```python
from build123d import *

# Parameters (mm, degrees)
SKETCH1_R           = 8
BOSS_EXTRUDE1_DEPTH = 6
SKETCH2_R           = 9.5
BOSS_EXTRUDE2_DEPTH = 2
SKETCH3_R           = 6.25
SKETCH3_R_2         = 4.25
CUT_EXTRUDE1_DEPTH  = 5
CHAMFER1_SIZE       = 1
CHAMFER2_SIZE       = 1
CUT_EXTRUDE2_DEPTH  = 16.636495771
CUT_EXTRUDE3_DEPTH  = 0.5


with BuildPart() as part:
    # Sketch1 → Boss-Extrude1 (new body)
    with BuildSketch(Plane(origin=(0, 0, 0), x_dir=(1, 0, 0), z_dir=(0, 1, 0))):
        with Locations(Location((0, 0, 0), (0, 0, 270))):
            Circle(SKETCH1_R)
    extrude(amount=BOSS_EXTRUDE1_DEPTH)

    # Sketch2 → Boss-Extrude2 (add)
    with BuildSketch(Plane.XZ):
        with Locations(Location((0, 0, 0), (0, 0, 270))):
            Circle(SKETCH2_R)
    extrude(amount=BOSS_EXTRUDE2_DEPTH)

    # Sketch3 → Cut-Extrude1 (cut)
    with BuildSketch(Plane.XZ.offset(2)):
        with Locations(Location((0, 0, 0), (0, 0, 270))):
            Circle(SKETCH3_R)
        with Locations(Location((0, 0, 0), (0, 0, 270))):
            Circle(SKETCH3_R_2, mode=Mode.SUBTRACT)
    extrude(amount=-CUT_EXTRUDE1_DEPTH, mode=Mode.SUBTRACT)

    # Chamfer1
    chamfer1_edges = [part.edges().sort_by_distance(p)[0] for p in [
        (0, -2, 6.25),
    ]]
    chamfer(chamfer1_edges, length=CHAMFER1_SIZE)

    # Chamfer2
    chamfer2_edges = [part.edges().sort_by_distance(p)[0] for p in [
        (0, -2, 4.25),
    ]]
    chamfer(chamfer2_edges, length=CHAMFER2_SIZE)

    # Sketch5 → Cut-Extrude2 (cut, through all)
    with BuildSketch(Plane.XZ.offset(2)):
        with BuildLine():
            Line((-1.25, -16.547716643), (1.25, -16.547716643))
            Line((1.25, -16.547716643), (1.25, -7.901740315))
            ThreePointArc((1.25, -7.901740315), (0, -8), (-1.25, -7.901740315))
            Line((-1.25, -7.901740315), (-1.25, -16.547716643))
        make_face()
    extrude(amount=-CUT_EXTRUDE2_DEPTH, mode=Mode.SUBTRACT)

    # Sketch6 → Cut-Extrude3 (cut)
    with BuildSketch(Plane(origin=(0, 6, 0), x_dir=(1, 0, 0), z_dir=(0, 1, 0))):
        with BuildLine():
            Line((0.5, 6.136828952), (0.5, 2.523425086))
            ThreePointArc((0.5, 2.523425086), (0, 2.023425086), (-0.5, 2.523425086))
            Line((-0.5, 2.523425086), (-0.5, 6.136828952))
            ThreePointArc((-0.5, 6.136828952), (0, 6.636828952), (0.5, 6.136828952))
        make_face()
        with BuildLine():
            ThreePointArc((-2.75, 4.763139721), (0, -5.5), (2.75, 4.763139721))
            ThreePointArc((2.75, 4.763139721), (2.066987298, 4.580127019), (2.25, 3.897114317))
            ThreePointArc((2.25, 3.897114317), (0, -4.5), (-2.25, 3.897114317))
            ThreePointArc((-2.25, 3.897114317), (-2.066987298, 4.580127019), (-2.75, 4.763139721))
        make_face()
    extrude(amount=-CUT_EXTRUDE3_DEPTH, mode=Mode.SUBTRACT)


solid = part.part
```
CAD build for the part. Positions are in the model's coordinates, mm. A direction names the side the tool comes from. Coordinates: 2 decimals unless noted, no trailing zeros. Write each loop counter-clockwise with the first axis right and the second up, starting at its lowest first coordinate (ties: lowest second). Pieces come first, ordered by that corner, then holes. Notation, with made-up numbers: (56.5, 72.5) -> (84.5, 72.5) arc R18 cw to (84.5, 96.5) -> close; hole circle Ø11 at (-21, 1). An arc over 180 degrees is marked (long way). Return JSON: item names as keys, results as strings. Group by question number.
Q1. Cut at B-B, the plane z = 0. Give the cut face in (x, y), then the cut area to 3 significant figures.
Q2. Pull direction Z, two halves, no side cores. Call faces 6 (the face through (1.25, -1, -9)), 7 (the face through (0.4, -0.99, 9.49)), 8 (the face through (1.88, 0.97, -5.96)): released by +Z, released by -Z, zero draft, split by the parting line, or undercut.
Q3. Cut at D-D, the plane y = 2. Give the cut face in (x, z), then the cut area to 3 significant figures.
Q4. Drill centre lines: line 1 (X direction, y = -0.1, z = 0); line 2 (X direction, y = 0.55, z = 0); line 3 (Z direction, x = 0, y = 5.85). Where is each one in solid material? Low to high.
Q5. Cut at A-A, the plane y = -0.25. Give the cut face in (x, z).
Q6. Which spindle directions (+Z, -Z, +X, -X, +Y, -Y) get a long thin tool onto all of the face, cutting with end or side? Do faces 1 (the face through (4.214, 0.972, 0.553)), 2 (the face through (0, 6, 0)), 3 (the face through (0, 5.5, 5)), 4 (the face through (0, -2, 0)), 5 (the face through (-1.25, -1, -9)). Say none if no direction does.
Q7. Cut at C-C, the plane x = 0. Give the cut face in (y, z).
Q8. Flat gauge pins, fed straight in: pin 1 (0.6 mm diameter, centred on y = 5.5, z = -5, fed in from -X); pin 2 (0.5 mm diameter, centred on y = -1, z = -9, fed in from -X); pin 3 (1.5 mm diameter, centred on x = -3, y = -1, fed in from +Z). Where does each tip first touch, or does it go through?
Returned:
{
 "1": {"outline": "(-9.5, -2) -> (-7.25, -2) -> (-6.25, -1) -> (-6.25, 3) -> (-4.25, 3) -> (-4.25, -1) -> (-3.25, -2) -> (3.25, -2) -> (4.25, -1) -> (4.25, 3) -> (6.25, 3) -> (6.25, -1) -> (7.25, -2) -> (9.5, -2) -> (9.5, 0) -> (8, 0) -> (8, 6) -> (5.5, 6) -> (5.5, 5.5) -> (4.5, 5.5) -> (4.5, 6) -> (-4.5, 6) -> (-4.5, 5.5) -> (-5.5, 5.5) -> (-5.5, 6) -> (-8, 6) -> (-8, 0) -> (-9.5, 0) -> close", "area": "111 mm2"},
 "2": {"face 6": "zero draft", "face 7": "split by the parting line", "face 8": "undercut"},
 "3": {"outline": "circle Ø16 at (0, 0); circle Ø8.5 at (0, 0); hole circle Ø12.5 at (0, 0)", "area": "135 mm2"},
 "4": {"line 1": "x = -9.5 to -6.25, -4.25 to 4.25, 6.25 to 9.5", "line 2": "x = -8 to -6.25, -4.25 to 4.25, 6.25 to 8", "line 3": "z = -8 to -6.64, -2.02 to 4.5, 5.5 to 8"},
 "5": {"outline": "circle Ø8.5 at (0, 0); (-1.25, -9.42) -> (-1.25, -7.9) arc R8 ccw to (1.25, -7.9) -> (1.25, -9.42) arc R9.5 ccw (long way) to start; hole circle Ø12.5 at (0, 0)"},
 "6": {"face 1": "-Y", "face 2": "+Z, -Z, +X, -X, +Y", "face 3": "+Y", "face 4": "+Z, -Z, +X, -X, -Y", "face 5": "-Z, +Y, -Y"},
 "7": {"outline": "(-2, -8) -> (6, -8) -> (6, -6.64) -> (5.5, -6.64) -> (5.5, -2.02) -> (6, -2.02) -> (6, 4.5) -> (5.5, 4.5) -> (5.5, 5.5) -> (6, 5.5) -> (6, 8) -> (0, 8) -> (0, 9.5) -> (-2, 9.5) -> (-2, 7.25) -> (-1, 6.25) -> (3, 6.25) -> (3, 4.25) -> (-1, 4.25) -> (-2, 3.25) -> (-2, -3.25) -> (-1, -4.25) -> (3, -4.25) -> (3, -6.25) -> (-1, -6.25) -> (-2, -7.25) -> close"},
 "8": {"pin 1": "stops at x = -6.47", "pin 2": "stops at x = -3.7", "pin 3": "stops at z = 9.23"}
}
